Could you check a few things on this drawing? It's one solid part, dimensions in mm from its lowest x, y, z. A direction names the side the tool comes from. Give positions to 0.01 mm unless a question says otherwise; leave off trailing zeros. Loops run counter-clockwise (first coordinate to the right, second up) from the corner with the lowest first, then second, coordinate; pieces in that order, holes last. Notation, with made-up numbers: M 5.25,16 L 48.25,16 A30 ccw 48.25,45 Z; hole C -24.5,-4 d5. An arc over 180 degrees is marked long. Answer in a Markdown table with one row per item. Add a question column.
1. I'm going to push flat-ended pins straight in: pin 1 Ø1.5 at (x, z) = (22, 5.5) entering from -Y; pin 2 Ø14.5 at (y, z) = (22, 32) entering from -X; pin 3 Ø2.5 at (y, z) = (23, 4.5) entering from +X; pin 4 Ø3 at (x, y) = (15.5, 4.5) entering from -Z. Where does each tip first touch, or does it pass through?
2. I need wall thicknesses on line 1 along X through (y, z) = (14, 76); line 2 along Z through (x, y) = (13.75, 17.75); line 3 along Z through (x, y) = (9.25, 9). Which ranges of each line are inside material? Lowest first, please. Write a range as from..to.
3. If we section it at B-B on y = 7.25: List the corners of the cut face in (x, z) for me, then the cut area to 3 significant figures.
4. If we section it at C-C on z = 52: List the corners of the cut face in (x, y) for me, then the cut area to 3 significant figures.
5. Which directions (+Z, -Z, +X, -X, +Y, -Y) give clear straight access to the entire face, cutting with the end or side of a thin tool? Please do the marked faces 1, 2 and 3.
6. If we section it at A-A on x = 7.75: List the corners of the cut face in (y, z) for me, then the cut area to 3 significant figures.
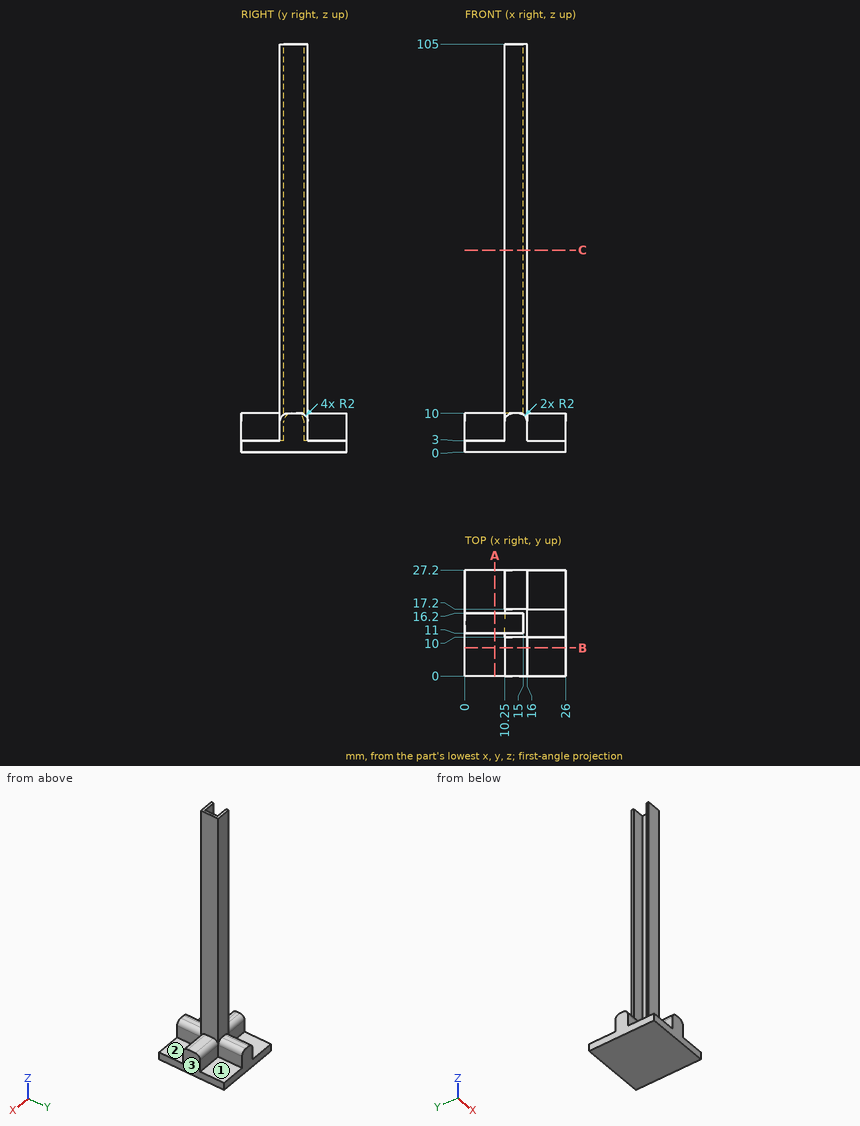
Results:
| question | item | result |
|---|---|---|
| 1 | pin 1 | y = 10 |
| 1 | pin 2 | x = 10.25 |
| 1 | pin 3 | x = 16 |
| 1 | pin 4 | z = 0 |
| 2 | line 1 | 15..16 |
| 2 | line 2 | 0..10 |
| 2 | line 3 | 0..3 |
| 3 | outline | M 0,0 L 26,0 L 26,3 L 16,3 L 16,8 A2 ccw 14,10 L 12.25,10 A2 ccw 10.25,8 L 10.25,3 L 0,3 Z |
| 3 | area | 117 mm2 |
| 4 | outline | M 10.25,10 L 16,10 L 16,17.2 L 10.25,17.2 L 10.25,16.2 L 15,16.2 L 15,11 L 10.25,11 Z |
| 4 | area | 16.7 mm2 |
| 5 | face 1 | +Z, +X, +Y |
| 5 | face 2 | +Z, +X, -Y |
| 5 | face 3 | +Z, -Z, +X, +Y, -Y |
| 6 | outline | M 0,0 L 27.2,0 L 27.2,3 L 16.2,3 L 16.2,8 A2 ccw 14.2,10 L 13,10 A2 ccw 11,8 L 11,3 L 0,3 Z |
| 6 | area | 116 mm2 |
